Design review of the part built by this model. Coordinates are the model's own, in mm. Face numbers are marked on the shaded views. A direction names the side the tool comes from. Give positions to 0.01 mm unless a question says otherwise; leave off trailing zeros. Loops run counter-clockwise (first coordinate to the right, second up) from the corner with the lowest first, then second, coordinate; pieces in that order, holes last. Notation, with made-up numbers: (47.25, 50) -> (91.25, 50) arc R8 ccw to (91.25, 60) -> close; hole circle Ø3 at (74.25, 17.5). An arc over 180 degrees is marked (long way). Answer as CSV lines item,"result".
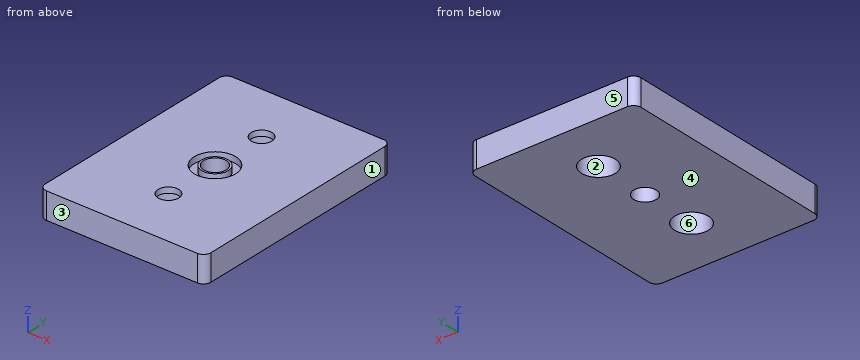
from build123d import *

# Parameters (mm, degrees)
F0_W           = 44
F0_H           = 60
F1_DEPTH       = 7
F2_R           = 2
F3_R           = 3
F4_DEPTH       = 7.001
F5_D           = 5.5
F5_CBORE_D     = 9
F5_CBORE_DEPTH = 5.5
F6_R           = 5.5
F6_R_2         = 3.5
F7_DEPTH       = 1.65


with BuildPart() as f1:
    # F0 (on Top) → F1 (new body)
    with BuildSketch(Plane.XY):
        Rectangle(F0_W, F0_H)
    extrude(amount=F1_DEPTH)

    # F2
    f2_edges = [f1.edges().sort_by_distance(p)[0] for p in [
        (-22, -30, 3.5),
        (22, -30, 3.5),
        (22, 30, 3.5),
        (-22, 30, 3.5),
    ]]
    fillet(f2_edges, radius=F2_R)

    # F3 (on face) → F4 (cut, through all)
    with BuildSketch(Plane(origin=(0, 0, 0), x_dir=(1, 0, 0), z_dir=(0, 0, -1))):
        Circle(F3_R)
    extrude(amount=-F4_DEPTH, mode=Mode.SUBTRACT)

    # F5 (through all)
    with Locations(Plane(origin=(0, 0, 0), x_dir=(1, 0, 0), z_dir=(0, 0, -1))):
        with Locations((0, -15), (0, 15)):
            CounterBoreHole(F5_D / 2, F5_CBORE_D / 2, F5_CBORE_DEPTH)

    # F6 (on face) → F7 (cut)
    with BuildSketch(Plane.XY.offset(7)):
        Circle(F6_R)
        Circle(F6_R_2, mode=Mode.SUBTRACT)
    extrude(amount=-F7_DEPTH, mode=Mode.SUBTRACT)


solid = f1.part
Q1. We need section B-B, the plane y = 0. State the section outline as (x, z) points, and give its area (3 significant figures).
Filled sheet:
outline,"(-22, 0) -> (-3, 0) -> (-3, 7) -> (-3.5, 7) -> (-3.5, 5.35) -> (-5.5, 5.35) -> (-5.5, 7) -> (-22, 7) -> close; (3, 0) -> (22, 0) -> (22, 7) -> (5.5, 7) -> (5.5, 5.35) -> (3.5, 5.35) -> (3.5, 7) -> (3, 7) -> close"
area,"259 mm^2"
Q2. We need section D-D, the plane y = 15. State the section outline as (x, z) points, and give its area (3 significant figures).
Filled sheet:
outline,"(-22, 0) -> (-4.5, 0) -> (-4.5, 5.5) -> (-2.75, 5.5) -> (-2.75, 7) -> (-22, 7) -> close; (2.75, 5.5) -> (4.5, 5.5) -> (4.5, 0) -> (22, 0) -> (22, 7) -> (2.75, 7) -> close"
area,"250 mm^2"
Q3. We need section A-A, the plane x = 0. State how many separate pieces and enclosed holes the cut face has, and give its area (3 significant figures).
Filled sheet:
separate pieces,"4"
enclosed holes,"0"
area,"256 mm^2"
Q4. We need section C-C, the plane z = 3.25. State the section outline as (x, y) points.
Filled sheet:
outline,"(-22, -28) arc R2 ccw to (-20, -30) -> (20, -30) arc R2 ccw to (22, -28) -> (22, 28) arc R2 ccw to (20, 30) -> (-20, 30) arc R2 ccw to (-22, 28) -> close; hole circle Ø9 at (0, -15); hole circle Ø9 at (0, 15); hole circle Ø6 at (0, 0)"
Q5. Clearance check with a flat-ended pin moving along its axis: pin 1 Ø4.5 at (x, y) = (0.5, 14) entering from -Z. State where the tip first meets the part, or that it passes through.
Filled sheet:
pin 1,"stops at z = 5.5"
Q6. The part is to be moulded in two halves that separate along Y. For the marked faces 3, 4, 5 and 6, say which applies: pulls with the +Y half, pulls with the -Y half, needs draft (parallel to the pull), parting line crosses it, or undercut.
Filled sheet:
face 3,"pulls with the -Y half"
face 4,"needs draft"
face 5,"pulls with the +Y half"
face 6,"undercut"
Q7. For the marked faces 1 and 2, list the 3-axis set-ups (+Z, -Z, +X, -X, +Y, -Y) from which the entire face can be reached by the end or side of a thin tool; tool diameter is ignored.
Filled sheet:
face 1,"+Z, -Z, +X, +Y, -Y"
face 2,"-Z"
Q8. To check wall thickness, follow probe 1 along Y at (x, z) = (0, 5.95); probe 2 along Y at (x, z) = (0, 3.7); probe 3 along X at (y, z) = (15, 6). State the ranges of each line that lie inside material, in increasing order. Write a range as from..to.
Filled sheet:
probe 1,"y = -30..-17.75, -12.25..-5.5, -3.5..-3, 3..3.5, 5.5..12.25, 17.75..30"
probe 2,"y = -30..-19.5, -10.5..-3, 3..10.5, 19.5..30"
probe 3,"x = -22..-2.75, 2.75..22"
